Autodesk Inventor part; units mm, degrees
ref_plane "YZ Plane" through (0, 0, 0) normal (1, 0, 0) x (0, 1, 0)
ref_plane "XZ Plane" through (0, 0, 0) normal (0, 1, 0) x (-1, 0, 0)
ref_plane "XY Plane" through (0, 0, 0) normal (0, 0, 1) x (1, 0, 0)
sketch "Sketch1" plane through (0, 0, 0) normal (0, 0, 1) x (1, 0, 0)
  point P0 (0, 0)
sketch "Sketch2" plane through (0, 0, 0) normal (0, 0, 1) x (1, 0, 0)
  line L0 (0, 0) -> (15.875, 0)
  line L1 (15.875, 0) -> (15.875, 12.7)
  line L2 (15.875, 12.7) -> (0, 12.7)
  line L3 (0, 12.7) -> (0, 0)
  dimension "d0" = 15.875
  dimension "d1" = 12.7
extrude "Extrusion1" add sketch "Sketch2" along normal blind 12.7
sketch "Sketch3" plane through (0, 0, 12.7) normal (0, 0, 1) x (1, 0, 0)
  line L0 (0, 12.7) -> (0, 0)
  line L1 (0, 0) -> (2.032, 0)
  line L2 (0, 0) -> (15.875, 0)
  line L3 (2.032, 2.413) -> (14.097, 2.413)
  line L4 (14.097, 2.413) -> (14.097, 8.89)
  line L5 (14.097, 8.89) -> (2.032, 8.89)
  line L6 (2.032, 8.89) -> (2.032, 2.413)
extrude "Extrusion2" cut sketch "Sketch3" against normal blind 10.16
sketch "Sketch4" plane through (0, 0, 12.7) normal (0, 0, 1) x (1, 0, 0)
  line L0 (2.032, 8.89) -> (14.097, 8.89)
  line L1 (11.049, 8.89) -> (11.049, 10.668)
  line L2 (11.049, 10.668) -> (4.826, 10.668)
  line L3 (4.826, 10.668) -> (4.826, 8.89)
  line L4 (11.049, 8.89) -> (4.826, 8.89)
  point P0 (0, 0)
  dimension "d13" = 3.048
  dimension "d16" = 6.223
extrude "Extrusion3" cut sketch "Sketch4" against normal blind 10.16
sketch "Sketch5" plane through (0, 0, 12.7) normal (0, 0, 1) x (1, 0, 0)
  line L0 (11.049, 10.668) -> (11.049, 8.89)
  line L1 (4.826, 10.668) -> (11.049, 10.668)
  line L2 (9.779, 10.668) -> (9.779, 12.446)
  line L3 (9.779, 12.446) -> (6.096, 12.446)
  line L4 (6.096, 12.446) -> (6.096, 10.668)
  line L5 (6.096, 10.668) -> (9.779, 10.668)
  point P0 (0, 0)
extrude "Extrusion4" cut sketch "Sketch5" against normal blind 10.16
sketch "Sketch6" plane through (0, 0, 12.7) normal (0, 0, 1) x (1, 0, 0)
  line L0 (14.097, 2.413) -> (2.032, 2.413)
  line L1 (14.097, 8.89) -> (14.097, 2.413)
  line L2 (14.097, 4.953) -> (15.367, 4.953)
  line L3 (15.367, 4.953) -> (15.367, 7.493)
  line L4 (15.367, 7.493) -> (14.097, 7.493)
  line L5 (14.097, 7.493) -> (14.097, 4.953)
  line L6 (2.032, 2.413) -> (2.032, 8.89)
  line L7 (2.032, 4.953) -> (0.762, 4.953)
  line L8 (0.762, 4.953) -> (0.762, 7.493)
  line L9 (0.762, 7.493) -> (2.032, 7.493)
  line L10 (2.032, 7.493) -> (2.032, 4.953)
  point P0 (0, 0)
extrude "Extrusion5" cut sketch "Sketch6" against normal blind 10.16
sketch "Sketch7" plane through (0, 0, 12.7) normal (0, 0, 1) x (1, 0, 0)
  circle A0 centre (3.0514, 10.3254) radius 0.508
  point P0 (0, 0)
  dimension "d33" = 1.016
extrude "Extrusion6" cut sketch "Sketch7" against normal blind 10.16
properties part number "Ethernet Port" material "Acetal Resin, White"
Here's how the part is built. I have some questions about the finished solid (model axes, mm). A direction names the side the tool comes from. Give positions to 0.01 mm unless a question says otherwise; leave off trailing zeros. Loops run counter-clockwise (first coordinate to the right, second up) from the corner with the lowest first, then second, coordinate; pieces in that order, holes last. Notation, with made-up numbers: (70, -31.75) -> (94, -31.75) arc R36 ccw to (94, 7.25) -> close; hole circle Ø3 at (85.5, 46.5). An arc over 180 degrees is marked (long way). Answer as a JSON object with one key per item and string values. Group by question number.
Item 1: Will this pin go through, and if not, where does the flat tip stop? pin 1 (1.5 mm diameter, centred on x = 10.5, y = 4.5, fed in from +Z).
Item 2: Imagine slicing it at B-B on x = 6.75. Write out the boundary of the cut face in (y, z), then the cut area to 3 significant figures.
Item 3: I need wall thicknesses on L1, parallel to X at y = 5, z = 11.75 (3 decimals); L2, parallel to Y at x = 7.25, z = 5.25; L3, parallel to X at y = 10, z = 11.5 (1 decimal). Which ranges of each line are inside material? Lowest first, please.
Item 4: On a 3-axis mill with a long thin cutter (end or side, diameter ignored), from which of +Z, -Z, +X, -X, +Y, -Y can I reach the whole of each face in a straight line? I mean faces 3 (the flat face through (8, 6, 0)), 4 (the flat face through (15, 4.953, 8)). Say none if no direction works.
Item 5: Thinking about a two-plate mould opening in X: for faces 1 (the flat face through (1, 7.493, 8)), 2 (the flat face through (8, 0, 6)), which applies, pulls with the +X half, pulls with the -X half, needs draft (parallel to the pull), parting line crosses it, or undercut?
Item 6: Imagine slicing it at A-A on y = 7. Write out the boundary of the cut face in (x, z) (3 decimals), then the cut area to 3 significant figures.
Item 7: Imagine slicing it at C-C on z = 11.25. Write out the boundary of the cut face in (x, y) (3 decimals).
Answer list:
{
 "1": {"pin 1": "stops at z = 2.54"},
 "2": {"outline": "(0, 0) -> (12.7, 0) -> (12.7, 12.7) -> (12.45, 12.7) -> (12.45, 2.54) -> (2.41, 2.54) -> (2.41, 12.7) -> (0, 12.7) -> close", "area": "59.4 mm2"},
 "3": {"L1": "x = 0 to 0.762, 15.367 to 15.875", "L2": "y = 0 to 2.41, 12.45 to 12.7", "L3": "x = 0 to 2.7, 3.4 to 4.8, 11 to 15.9"},
 "4": {"face 3": "-Z, +X, -X, +Y, -Y", "face 4": "+Z"},
 "5": {"face 1": "undercut", "face 2": "needs draft"},
 "6": {"outline": "(0, 0) -> (15.875, 0) -> (15.875, 12.7) -> (15.367, 12.7) -> (15.367, 2.54) -> (0.762, 2.54) -> (0.762, 12.7) -> (0, 12.7) -> close", "area": "53.2 mm2"},
 "7": {"outline": "(0, 0) -> (15.875, 0) -> (15.875, 12.7) -> (0, 12.7) -> close; hole (0.762, 4.953) -> (2.032, 4.953) -> (2.032, 2.413) -> (14.097, 2.413) -> (14.097, 4.953) -> (15.367, 4.953) -> (15.367, 7.493) -> (14.097, 7.493) -> (14.097, 8.89) -> (11.049, 8.89) -> (11.049, 10.668) -> (9.779, 10.668) -> (9.779, 12.446) -> (6.096, 12.446) -> (6.096, 10.668) -> (4.826, 10.668) -> (4.826, 8.89) -> (2.032, 8.89) -> (2.032, 7.493) -> (0.762, 7.493) -> close; hole circle Ø1.016 at (3.051, 10.325)"}
}
